```python
from build123d import *

# Parameters (mm, degrees)
SKETCH_1_W          = 80
SKETCH_1_H          = 60
EXTRUDE_1_DEPTH     = 3
CUT_EXTRUDE_1_DEPTH = 3
EXTRUDE_2_DEPTH     = 20
SKETCH_4_W          = 6.5
SKETCH_4_H          = 45
CUT_EXTRUDE_2_DEPTH = 89.481636513
SKETCH_5_W          = 6
SKETCH_5_H          = 55
CUT_EXTRUDE_3_DEPTH = 1
SKETCH_7_W          = 20
SKETCH_7_H          = 8
SKETCH_7_W_2        = 12
CUT_EXTRUDE_4_DEPTH = 3
SKETCH_8_W          = 66
SKETCH_8_H          = 47
EXTRUDE_3_DEPTH     = 2
CUT_EXTRUDE_5_DEPTH = 56.901699437
CUT_EXTRUDE_6_DEPTH = 54.795910625
SKETCH_12_W         = 40
SKETCH_12_H         = 6
EXTRUDE_4_DEPTH     = 35
SKETCH_13_R         = 1.55
CUT_EXTRUDE_7_DEPTH = 76.59761901


with BuildPart() as part:
    # 草图1 → 凸台-拉伸1 (new body)
    with BuildSketch(Plane.XY):
        Rectangle(SKETCH_1_W, SKETCH_1_H)
    extrude(amount=EXTRUDE_1_DEPTH)

    # 草图2 → 切除-拉伸1 (cut)
    with BuildSketch(Plane.XY.offset(3)):
        Polygon((-12.5, -8.5), (-12.5, 8.5), (-12.5, 30), (12.5, 30), (12.5, 8.5), (12.5, -8.5), (12.5, -16), (-12.5, -16), align=None)
    extrude(amount=-CUT_EXTRUDE_1_DEPTH, mode=Mode.SUBTRACT)

    # 草图3 → 凸台-拉伸2 (add)
    with BuildSketch(Plane.XY.offset(3)):
        Polygon((-40, 30), (-35, 30), (-35, -25), (35, -25), (35, 30), (40, 30), (40, -30), (-40, -30), align=None)
    extrude(amount=EXTRUDE_2_DEPTH)

    # 草图4 → 切除-拉伸2 (cut, through all)
    with BuildSketch(Plane.ZY.offset(40)):
        with Locations((7.25, 2.5)):
            Rectangle(SKETCH_4_W, SKETCH_4_H)
    extrude(amount=-CUT_EXTRUDE_2_DEPTH, mode=Mode.SUBTRACT)

    # 草图5 → 切除-拉伸3 (cut)
    with BuildSketch(Plane.XY.offset(3)):
        with Locations((-30, 2.5)):
            Rectangle(SKETCH_5_W, SKETCH_5_H)
        with Locations((30, 2.5)):
            Rectangle(SKETCH_5_W, SKETCH_5_H)
    extrude(amount=-CUT_EXTRUDE_3_DEPTH, mode=Mode.SUBTRACT)

    # 草图7 → 切除-拉伸4 (cut)
    with BuildSketch(Plane.XY.offset(3)):
        with Locations((-15.5, -18)):
            Rectangle(SKETCH_7_W, SKETCH_7_H)
        with Locations((19.5, -18)):
            Rectangle(SKETCH_7_W_2, SKETCH_7_H)
    extrude(amount=-CUT_EXTRUDE_4_DEPTH, mode=Mode.SUBTRACT)

    # 草图8 → 凸台-拉伸3 (add)
    with BuildSketch(Plane.XY.offset(23)):
        Polygon((-40, 30), (-32, 30), (32, 30), (40, 30), (40, -30), (-40, -30), align=None)
        with Locations((0, 2)):
            Rectangle(SKETCH_8_W, SKETCH_8_H, mode=Mode.SUBTRACT)
    extrude(amount=EXTRUDE_3_DEPTH)

    # 草图9 → 切除-拉伸5 (cut, through all)
    with BuildSketch(Plane.XY.offset(25)):
        Polygon((-40, 30), (-37, 30), (-37, -26), (37, -26), (37, 30), (40, 30), (40, -30), (38, -30), (-38, -30), (-40, -30), align=None)
    extrude(amount=-CUT_EXTRUDE_5_DEPTH, mode=Mode.SUBTRACT)

    # 草图11 → 切除-拉伸6 (cut, through all)
    with BuildSketch(Plane.XY.offset(25)):
        with BuildLine():
            Line((-35.5, 30), (-37, 30))
            Line((-37, 30), (-37, 28.5))
            ThreePointArc((-37, 28.5), (-36.560660172, 29.560660172), (-35.5, 30))
        make_face()
        with BuildLine():
            Line((-37, -24.5), (-37, -26))
            Line((-37, -26), (-35.5, -26))
            ThreePointArc((-35.5, -26), (-36.560660172, -25.560660172), (-37, -24.5))
        make_face()
        with BuildLine():
            Line((37, -24.5), (37, -26))
            Line((37, -26), (35.5, -26))
            ThreePointArc((35.5, -26), (36.560660172, -25.560660172), (37, -24.5))
        make_face()
        with BuildLine():
            Line((35.5, 30), (37, 30))
            Line((37, 30), (37, 28.5))
            ThreePointArc((37, 28.5), (36.560660172, 29.560660172), (35.5, 30))
        make_face()
    extrude(amount=-CUT_EXTRUDE_6_DEPTH, mode=Mode.SUBTRACT)

    # 草图12 → 凸台-拉伸4 (add)
    with BuildSketch(Plane.XZ.offset(26)):
        with Locations((0, 22)):
            Rectangle(SKETCH_12_W, SKETCH_12_H)
    extrude(amount=EXTRUDE_4_DEPTH)

    # 草图13 → 切除-拉伸7 (cut, through all)
    with BuildSketch(Plane.XY.offset(25)):
        with Locations((-13, -39)):
            Circle(SKETCH_13_R)
        with Locations((13, -39)):
            Circle(SKETCH_13_R)
        with Locations((-13, -58.5)):
            Circle(SKETCH_13_R)
        with Locations((13, -58.5)):
            Circle(SKETCH_13_R)
        with BuildLine():
            Line((-4, -61), (4, -61))
            Line((4, -61), (4, -48.5))
            ThreePointArc((4, -48.5), (3.121320344, -46.378679656), (1, -45.5))
            Line((1, -45.5), (0, -45.5))
            Line((0, -45.5), (-1, -45.5))
            ThreePointArc((-1, -45.5), (-3.121320344, -46.378679656), (-4, -48.5))
            Line((-4, -48.5), (-4, -61))
        make_face()
        with BuildLine():
            Line((20, -58), (20, -61))
            Line((20, -61), (17, -61))
            ThreePointArc((17, -61), (19.121320344, -60.121320344), (20, -58))
        make_face()
        with BuildLine():
            Line((-20, -58), (-20, -61))
            Line((-20, -61), (-17, -61))
            ThreePointArc((-17, -61), (-19.121320344, -60.121320344), (-20, -58))
        make_face()
    extrude(amount=-CUT_EXTRUDE_7_DEPTH, mode=Mode.SUBTRACT)


solid = part.part
```
For this review, take the finished solid that the model builds, in its own axes (mm). A direction names the side the tool comes from. Round coordinates to 2 decimals unless told otherwise and drop trailing zeros. Order: outer loops, then holes, each group sorted by start corner. A loop starts at its lowest first (then second) coordinate and runs counter-clockwise, first axis right, second up.
Q1. We need section A-A, the plane x = 24. Give the boundary of the cut face in (y, z), plus the area to 3 significant figures.
Findings below:
outline: (-26, 0) - (-22, 0) - (-22, 3) - (-25, 3) - (-25, 23) - (-21.5, 23) - (-21.5, 25) - (-26, 25) - close; (-14, 0) - (30, 0) - (30, 3) - (-14, 3) - close; (25.5, 23) - (30, 23) - (30, 25) - (25.5, 25) - close
area: 182 mm2
Q2. Machinability: for faces 4 (the flat face through (18, 9, 3)), 5 (the flat face through (0, -21.5, 24)), 6 (the flat face through (0, -43, 19)), 7 (the cylindrical face through (-3.1, -46.36, 22.04)), which of the approach directions +Z, -Z, +X, -X, +Y, -Y give a long, thin tool a straight path to every point of the face, cutting with its end or side? Answer none if there is none.
Findings below:
face 4: +Y
face 5: +Z
face 6: -Z, +X, -X, -Y
face 7: +Z, -Z, -Y
Q3. Insertion check: P1, Ø3.5, axis at x = 6.5, z = 1, coming from the +Y side; P2, Ø10.5, axis at x = 9.5, y = -41.5, coming from the -Z side; P3, Ø0.9, axis at x = -11.5, z = 1, coming from the +Y side; P4, Ø2.5, axis at x = -13, y = -58.5, coming from the +Z side. Each pin has a flat end and moves straight along its axis. Give the tip position at first contact, or say it passes through.
Findings below:
P1: stops at y = -16
P2: stops at z = 19
P3: stops at y = -22
P4: passes through
Q4. We need section B-B, the plane y = 20. State how many separate pieces and enclosed holes the cut face has, plus the area to 3 significant figures.
Findings below:
separate pieces: 4
enclosed holes: 0
area: 205 mm2
Q5. We need section C-C, the plane z = 15.75. Give the boundary of the cut face in (x, y), plus the area to 3 significant figures.
Findings below:
outline: (-37, -24.5) arc R1.5 ccw to (-35.5, -26) - (35.5, -26) arc R1.5 ccw to (37, -24.5) - (37, 28.5) arc R1.5 ccw to (35.5, 30) - (35, 30) - (35, -25) - (-35, -25) - (-35, 30) - (-35.5, 30) arc R1.5 ccw to (-37, 28.5) - close
area: 292 mm2
Q6. Wall thickness on line 1 (Y direction, x = 13, z = 21.75); line 2 (Y direction, x = -13, z = 23.7); line 3 (Z direction, x = -21.5, y = -22.5): over which ranges is each line inside the solid? List them lowest first.
Findings below:
line 1: y = -61 to -60.05, -56.95 to -40.55, -37.45 to -25
line 2: y = -61 to -60.05, -56.95 to -40.55, -37.45 to -21.5, 25.5 to 30
line 3: z = 0 to 3, 23 to 25
Q7. We need section D-D, the plane y = -39. Give the boundary of the cut face in (x, z), plus the area to 3 significant figures.
Findings below:
outline: (-20, 19) - (-14.55, 19) - (-14.55, 25) - (-20, 25) - close; (-11.45, 19) - (11.45, 19) - (11.45, 25) - (-11.45, 25) - close; (14.55, 19) - (20, 19) - (20, 25) - (14.55, 25) - close
area: 203 mm2
Q8. Mouldability with a two-part tool opening along Y and no side actions: class faces 1 (the flat face through (-36, 2, 4)), 2 (the flat face through (-5.5, -19, 2)), 3 (the flat face through (0, 30, 24)) as pulls with the +Y half, pulls with the -Y half, needs draft (parallel to the pull), parting line crosses it, or undercut.
Findings below:
face 1: undercut
face 2: needs draft
face 3: pulls with the +Y half
